Geometry check sheet. Reference: the model listing, model coordinates, mm. Face numbers are marked on the shaded views. A direction names the side the tool comes from. Give positions to 0.01 mm unless a question says otherwise; leave off trailing zeros. Order: outer loops, then holes, each group sorted by start corner. A loop starts at its lowest first (then second) coordinate and runs counter-clockwise, first axis right, second up.
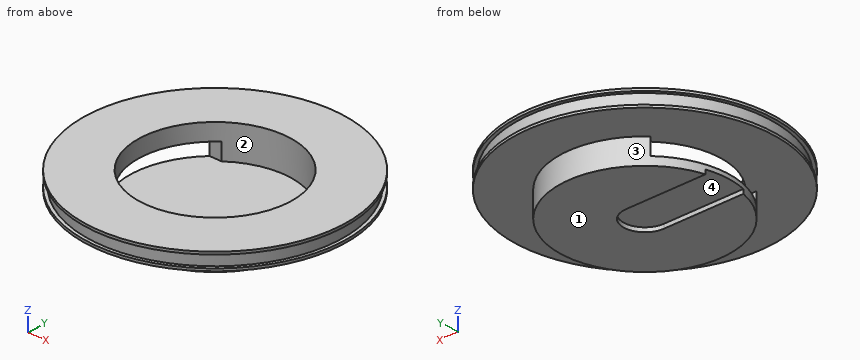
Autodesk Inventor part; units mm, degrees
ref_plane "YZ Plane" through (0, 0, 0) normal (1, 0, 0) x (0, 1, 0)
ref_plane "XZ Plane" through (0, 0, 0) normal (0, 1, 0) x (-1, 0, 0)
ref_plane "XY Plane" through (0, 0, 0) normal (0, 0, 1) x (1, 0, 0)
sketch "Sketch1" plane through (0, 0, 0) normal (0, 0, 1) x (1, 0, 0)
  circle A0 centre (0, 0) radius 77
  dimension "d0" = 154
extrude "Extrusion1" add sketch "Sketch1" along normal blind 1.5
sketch "Sketch2" plane through (0, 0, 1.5) normal (0, 0, 1) x (1, 0, 0)
  circle A0 centre (0, 0) radius 77
  circle A1 centre (0, 0) radius 75
  dimension "d4" = 150
extrude "Extrusion2" add sketch "Sketch2" along normal blind 7 contours A1
sketch "Sketch3" plane through (0, 0, 8.5) normal (0, 0, 1) x (1, 0, 0)
  circle A0 centre (0, 0) radius 77
extrude "Extrusion3" add sketch "Sketch3" along normal blind 1.5
sketch "Sketch5" plane through (0, 0, 0) normal (0, 0, -1) x (-1, 0, 0)
  circle A0 centre (0, 0) radius 77
  circle A1 centre (0, 0) radius 50
  dimension "d14" = 100
extrude "Extrusion5" add sketch "Sketch5" along normal blind 15 contours A1
sketch "Sketch6" plane through (0, 0, -15) normal (0, 0, -1) x (-1, 0, 0)
  circle A0 centre (0, 0) radius 50
  line L0 (48.4123, 12.5) -> (0, 12.5)
  arc A1 (0, 12.5) -> (0, -12.5) centre (0, 0) ccw
  line L1 (0, -12.5) -> (48.4123, -12.5)
  dimension "d18" = 25
extrude "Extrusion6" cut sketch "Sketch6" against normal blind 2.5 contours A0 L1 A1 L0 picked at (16.6667, 0)
sketch "Sketch7" plane through (0, 0, 10) normal (0, 0, 1) x (1, 0, 0)
  circle A0 centre (0, 0) radius 77
  circle A1 centre (0, 0) radius 45
  dimension "d22" = 90
extrude "Extrusion7" cut sketch "Sketch7" against normal blind 20 contours A1
sketch "Sketch8" plane through (0, 0, -10) normal (0, 0, 1) x (1, 0, 0)
  circle A0 centre (0, 0) radius 45
  line L0 (0, 35) -> (-105.83, 35)
  line L1 (-105.83, 35) -> (-105.83, -35)
  line L2 (-105.83, -35) -> (0, -35)
  arc A1 (0, -35) -> (0, 35) centre (0, 0) ccw
  dimension "d26" = 70
extrude "Extrusion8" cut sketch "Sketch8" along normal up to surface (10 mm away) contours L0 A1 L2 A0 | A0 L2 L1 L0 picked at (-14.9265, 1.4828)
properties part number "proximal drive pulley"
Q1. Cross-section at A-A, the plane y = 0. Record the boundary of the cut face in (x, z).
Q2. Cross-section at D-D, the plane x = 34.5. Record the boundary of the cut face in (y, z), and give its area (3 significant figures).
Q3. Access from +Z, -Z, +X, -X, +Y, -Y to the whole of each face (thin tool, end or side, straight path). Record for the marked faces 1, 2, 3 and 4.
Q4. Thickness scan on L1, parallel to Z at x = -39, y = 28.5; L2, parallel to Y at x = 0, z = 5.25; L3, parallel to Y at x = 0, z = -3.75. Record the ranges inside material, lowest first.
Q5. Gauge pin test, flat ends, axial feed: P1, Ø8, axis at x = 34, z = -2.5, coming from the -Y side; P2, Ø3, axis at y = 28.5, z = -5, coming from the -X side; P3, Ø8, axis at x = -28.5, z = -8, coming from the +Y side. Record the tip position at first contact, or that the pin passes through.
Q6. Cross-section at C-C, the plane y = 25. Record the boundary of the cut face in (x, z).
Q7. Cross-section at B-B, the plane x = -40. Record the boundary of the cut face in (y, z).
Answers follow:
1. outline: (-77, 0) - (-45, 0) - (-45, 10) - (-77, 10) - (-77, 8.5) - (-75, 8.5) - (-75, 1.5) - (-77, 1.5) - close; (-50, -12.5) - (12.5, -12.5) - (12.5, -15) - (50, -15) - (50, 0) - (77, 0) - (77, 1.5) - (75, 1.5) - (75, 8.5) - (77, 8.5) - (77, 10) - (45, 10) - (45, -10) - (-50, -10) - close
2. outline: (-68.84, 0) - (-36.19, 0) - (-36.19, -15) - (36.19, -15) - (36.19, 0) - (68.84, 0) - (68.84, 1.5) - (66.59, 1.5) - (66.59, 8.5) - (68.84, 8.5) - (68.84, 10) - (28.89, 10) - (28.89, -10) - (-28.89, -10) - (-28.89, 10) - (-68.84, 10) - (-68.84, 8.5) - (-66.59, 8.5) - (-66.59, 1.5) - (-68.84, 1.5) - close
2. area: 1,280 mm2
3. face 1: -Z, +X, -X, +Y, -Y
3. face 2: +Z
3. face 3: -Z
3. face 4: -Z, -X
4. L1: z = -15 to -10, 0 to 10
4. L2: y = -75 to -45, 45 to 75
4. L3: y = -50 to -45, 45 to 50
5. P1: stops at y = -70.54
5. P2: stops at x = 33.54
5. P3: stops at y = 43.59
6. outline: (-72.83, 0) - (-37.42, 0) - (-37.42, 10) - (-72.83, 10) - (-72.83, 8.5) - (-70.71, 8.5) - (-70.71, 1.5) - (-72.83, 1.5) - close; (-43.3, -15) - (43.3, -15) - (43.3, 0) - (72.83, 0) - (72.83, 1.5) - (70.71, 1.5) - (70.71, 8.5) - (72.83, 8.5) - (72.83, 10) - (37.42, 10) - (37.42, -10) - (-43.3, -10) - close
7. outline: (-65.8, 0) - (-20.62, 0) - (-20.62, 10) - (-65.8, 10) - (-65.8, 8.5) - (-63.44, 8.5) - (-63.44, 1.5) - (-65.8, 1.5) - close; (-30, -15) - (-12.5, -15) - (-12.5, -12.5) - (12.5, -12.5) - (12.5, -15) - (30, -15) - (30, -10) - (-30, -10) - close; (20.62, 0) - (65.8, 0) - (65.8, 1.5) - (63.44, 1.5) - (63.44, 8.5) - (65.8, 8.5) - (65.8, 10) - (20.62, 10) - close
